Check sheet for the modelled part. Datum: model origin and axes. Units: mm. Face numbers are marked on the shaded views. A direction names the side the tool comes from. Round coordinates to 2 decimals unless told otherwise and drop trailing zeros. Loops run counter-clockwise (first coordinate to the right, second up) from the corner with the lowest first, then second, coordinate; pieces in that order, holes last. Notation, with made-up numbers: (-33, 16) -> (15, 16) arc R34 ccw to (15, 46) -> close; hole circle Ø7 at (49.25, 54.25). An arc over 180 degrees is marked (long way). One line per item, written item: value. Start each with the question number.
1. Cross-section at D-D on y = 24.5. Record the cut outline in (x, z), then the cut area to 3 significant figures.
2. Cross-section at A-A on x = 7. Record the cut outline in (y, z), then the cut area to 3 significant figures.
3. Go/stop test with flat-tipped pins: pin 1 (1.2 mm diameter, centred on x = -12, z = 0.5, fed in from +Y); pin 2 (4 mm diameter, centred on x = -9.5, y = 22, fed in from -Z); pin 3 (12 mm diameter, centred on x = -4, y = 3, fed in from +Z); pin 4 (1.6 mm diameter, centred on y = 6.5, z = 0.5, fed in from +X). Record where each tip stops, or that it passes through.
4. Release check for a two-part mould opening along Y. For the marked faces 5, 6 and 7 record: +Y half, -Y half, draft (parallel to the pull), parting line (faces both ways), or undercut.
5. Cross-section at C-C on z = 2.5. Count the separate pieces of the cut face and the enclosed holes in it, then the cut area to 3 significant figures.
6. Set-up check for the marked faces 1, 2, 3 and 4: record each of +Z, -Z, +X, -X, +Y, -Y from which the full face is reachable in a straight line by a thin tool's end or side.
7. Material ranges on L1, parallel to X at y = -3, z = 1.25; L2, parallel to Y at x = -14, z = 4.75; L3, parallel to Y at x = 32, z = 6, recorded low to high.
8. Cross-section at B-B on y = -13. Record the cut outline in (x, z), then the cut area to 3 significant figures.
from build123d import *

# Parameters (mm, degrees)
PAD_DEPTH       = 12.5
POCKET_DEPTH    = 11
POCKET001_DEPTH = 1.5
SKETCH052_W     = 7
SKETCH052_H     = 1
PAD001_DEPTH    = 1
CHAMFER_SIZE    = 0.5
SKETCH053_W     = 7
SKETCH053_H     = 1
PAD002_DEPTH    = 1
CHAMFER001_SIZE = 0.5
SKETCH054_W     = 7
SKETCH054_H     = 1
PAD003_DEPTH    = 1
CHAMFER002_SIZE = 0.5
SKETCH055_W     = 7
SKETCH055_H     = 1
PAD004_DEPTH    = 1
CHAMFER003_SIZE = 0.5
SKETCH056_W     = 1.5
SKETCH056_H     = 12
POCKET002_DEPTH = 12.5
SKETCH057_W     = 18
SKETCH057_H     = 1.5
POCKET003_DEPTH = 11
PAD005_DEPTH    = 12.5
POCKET004_DEPTH = 20
POCKET005_DEPTH = 11
SKETCH063_R     = 1.5
POCKET006_DEPTH = 20
POCKET007_DEPTH = 17
POCKET008_DEPTH = 11
PAD006_DEPTH    = 11
PAD007_DEPTH    = 1.5


with BuildPart() as part:
    # Sketch001 → Pad (new body)
    with BuildSketch(Plane.XY):
        Polygon((-22.5, 18.12132), (-18.12132, 22.5), (18.12132, 22.5), (22.5, 18.12132), (22.5, -18.12132), (18.12132, -22.5), (-18.12132, -22.5), (-22.5, -18.12132), align=None)
    extrude(amount=PAD_DEPTH)

    # Sketch002 (on Face10 of Pad) → Pocket (cut)
    with BuildSketch(Plane.XY.offset(12.5)):
        Polygon((-21, 17.5), (-17.5, 21), (17.5, 21), (21, 17.5), (21, -17.5), (17.5, -21), (-17.5, -21), (-21, -17.5), align=None)
    extrude(amount=-POCKET_DEPTH, mode=Mode.SUBTRACT)

    # Sketch003 (on Face19 of Pocket) → Pocket001 (cut)
    with BuildSketch(Plane.XY.offset(1.5)):
        Polygon((-16.257359, 18), (-18, 16.257359), (-18, 1.5), (-1.5, 1.5), (-1.5, 18), align=None)
        Polygon((-18, -16.257359), (-16.257359, -18), (-1.5, -18), (-1.5, -1.5), (-18, -1.5), align=None)
        Polygon((16.257359, -18), (18, -16.257359), (18, -1.5), (1.5, -1.5), (1.5, -18), align=None)
        Polygon((18, 1.5), (18, 16.257359), (16.257359, 18), (1.5, 18), (1.5, 1.5), align=None)
    extrude(amount=-POCKET001_DEPTH, mode=Mode.SUBTRACT)

    # Sketch052 (on Face31 of Pocket001) → Pad001 (join)
    with BuildSketch(Plane(origin=(-19.25, 19.25, 0), x_dir=(0.707107, 0.707107, 0), z_dir=(0.707107, -0.707107, 0))):
        with Locations((0, 12)):
            Rectangle(SKETCH052_W, SKETCH052_H)
    extrude(amount=PAD001_DEPTH)

    # Chamfer
    chamfer_edges = [part.edges().sort_by_distance(p)[0] for p in [
        (-18.542893, 18.542893, 11.5),
    ]]
    chamfer(chamfer_edges, length=CHAMFER_SIZE)

    # Sketch053 (on Face8 of Chamfer) → Pad002 (join)
    with BuildSketch(Plane(origin=(19.25, 19.25, 0), x_dir=(0.707107, -0.707107, 0), z_dir=(-0.707107, -0.707107, 0))):
        with Locations((0, 12)):
            Rectangle(SKETCH053_W, SKETCH053_H)
    extrude(amount=PAD002_DEPTH)

    # Chamfer001
    chamfer001_edges = [part.edges().sort_by_distance(p)[0] for p in [
        (18.542893, 18.542893, 11.5),
    ]]
    chamfer(chamfer001_edges, length=CHAMFER001_SIZE)

    # Sketch054 (on Face28 of Chamfer001) → Pad003 (join)
    with BuildSketch(Plane(origin=(-19.25, -19.25, 0), x_dir=(-0.707107, 0.707107, 0), z_dir=(0.707107, 0.707107, 0))):
        with Locations((0, 12)):
            Rectangle(SKETCH054_W, SKETCH054_H)
    extrude(amount=PAD003_DEPTH)

    # Chamfer002
    chamfer002_edges = [part.edges().sort_by_distance(p)[0] for p in [
        (-18.542893, -18.542893, 11.5),
    ]]
    chamfer(chamfer002_edges, length=CHAMFER002_SIZE)

    # Sketch055 (on Face6 of Chamfer002) → Pad004 (join)
    with BuildSketch(Plane(origin=(19.25, -19.25, 0), x_dir=(-0.707107, -0.707107, 0), z_dir=(-0.707107, 0.707107, 0))):
        with Locations((0, 12)):
            Rectangle(SKETCH055_W, SKETCH055_H)
    extrude(amount=PAD004_DEPTH)

    # Chamfer003
    chamfer003_edges = [part.edges().sort_by_distance(p)[0] for p in [
        (18.542893, -18.542893, 11.5),
    ]]
    chamfer(chamfer003_edges, length=CHAMFER003_SIZE)

    # Sketch056 (on Face7 of Chamfer003) → Pocket002 (cut)
    with BuildSketch(Plane.XY.offset(12.5)):
        with Locations((-21.75, -1.5)):
            Rectangle(SKETCH056_W, SKETCH056_H)
    extrude(amount=-POCKET002_DEPTH, mode=Mode.SUBTRACT)

    # Sketch057 (on Face7 of Pocket002) → Pocket003 (cut)
    with BuildSketch(Plane.XY.offset(12.5)):
        with Locations((0, 21.75)):
            Rectangle(SKETCH057_W, SKETCH057_H)
    extrude(amount=-POCKET003_DEPTH, mode=Mode.SUBTRACT)

    # Sketch058 → Pad005 (join)
    with BuildSketch(Plane.XY):
        Polygon((22.5, 12.5), (34.5, 12.5), (34.5, 32.5), (18.12132, 32.5), (18.12132, 22.5), (22.5, 18.12132), align=None)
    extrude(amount=PAD005_DEPTH)

    # Sketch059 (on Face71 of Pad005) → Pocket004 (cut)
    with BuildSketch(Plane.XZ.offset(-12.5)):
        with BuildLine():
            ThreePointArc((29.5, 1.5), (34.5, 6.5), (29.5, 11.5))
            Line((29.5, 11.5), (29.5, 12.5))
            Line((29.5, 12.5), (35.5, 12.5))
            Line((35.5, 12.5), (35.5, 0))
            Line((35.5, 0), (29.5, 0))
            Line((29.5, 0), (29.5, 1.5))
        make_face()
    extrude(amount=-POCKET004_DEPTH, mode=Mode.SUBTRACT)

    # Sketch060 (on Face44 of Pocket004) → Pocket005 (cut)
    with BuildSketch(Plane.XY.offset(12.5)):
        Polygon((18.12132, 22.5), (18.12132, 32.5), (22.5, 32.5), (22.5, 29.3), (34.5, 29.3), (34.5, 15.7), (22.5, 15.7), (22.5, 18.12132), align=None)
    extrude(amount=-POCKET005_DEPTH, mode=Mode.SUBTRACT)

    # Sketch063 → Pocket006 (cut)
    with BuildSketch(Plane.XZ.offset(-12.5)):
        with Locations((29.5, 6.5)):
            Circle(SKETCH063_R)
    extrude(amount=-POCKET006_DEPTH, mode=Mode.SUBTRACT)

    # Sketch064 (on Face90 of Pocket006) → Pocket007 (cut)
    with BuildSketch(Plane.XZ.offset(-31)):
        with BuildLine():
            ThreePointArc((29.5, 1), (33.389087, 10.389087), (24, 6.5))
            Line((24, 6.5), (24, 0))
            Line((24, 0), (29.5, 0))
            Line((29.5, 0), (29.5, 1))
        make_face()
    extrude(amount=POCKET007_DEPTH, mode=Mode.SUBTRACT)

    # Sketch065 (on Face7 of Pocket007) → Pocket008 (cut)
    with BuildSketch(Plane.XY.offset(12.5)):
        Polygon((16.085786, -21), (14.585786, -22.5), (6.085786, -22.5), (4.585786, -21), align=None)
    extrude(amount=-POCKET008_DEPTH, mode=Mode.SUBTRACT)

    # Sketch066 (on Face75 of Pocket008) → Pad006 (join)
    with BuildSketch(Plane.XY.offset(1.5)):
        Polygon((18.12132, 32.5), (22.5, 32.5), (22.5, 29.3), align=None)
    extrude(amount=PAD006_DEPTH)

    # Sketch067 → Pad007 (join)
    with BuildSketch(Plane.XY):
        Polygon((18.12132, 32.5), (9, 22.5), (18.12132, 22.5), align=None)
    extrude(amount=PAD007_DEPTH)


solid = part.part
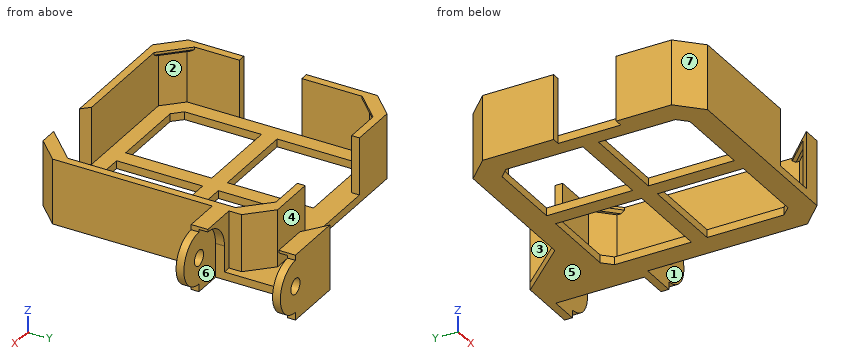
Taken from the geometry:
1. outline: (10.82, 0) -> (24, 0) -> (24, 1.5) -> (10.82, 1.5) -> close
1. area: 19.8 mm2
2. outline: (-22.5, 0) -> (-18, 0) -> (-18, 1.5) -> (-22.5, 1.5) -> close; (-1.5, 0) -> (1.5, 0) -> (1.5, 1.5) -> (-1.5, 1.5) -> close; (18, 0) -> (22.5, 0) -> (22.5, 1.5) -> (18, 1.5) -> close
2. area: 18.0 mm2
3. pin 1: stops at y = 22.5
3. pin 2: stops at z = 0
3. pin 3: stops at z = 1.5
3. pin 4: stops at x = 22.5
4. face 5: draft
4. face 6: undercut
4. face 7: -Y half
5. separate pieces: 4
5. enclosed holes: 0
5. area: 229 mm2
6. face 1: +Z, -Z, +X, -Y
6. face 2: none
6. face 3: +Z, -X
6. face 4: +Z, +X, -X, +Y
7. L1: x = -21 to -18, -1.5 to 1.5, 18 to 22.5
7. L2: y = -22.5 to -21, 21 to 22.5
7. L3: y = 12.5 to 14, 31 to 32.5
8. outline: (-22.5, 0) -> (-18, 0) -> (-18, 1.5) -> (-21, 1.5) -> (-21, 12.5) -> (-22.5, 12.5) -> close; (-1.5, 0) -> (1.5, 0) -> (1.5, 1.5) -> (-1.5, 1.5) -> close; (18, 0) -> (22.5, 0) -> (22.5, 12.5) -> (21, 12.5) -> (21, 1.5) -> (18, 1.5) -> close
8. area: 51.0 mm2
